from build123d import *

# Parameters (mm, degrees)
SKETCH1_R           = 3.4
SKETCH1_R_2         = 2.1
BOSS_EXTRUDE1_DEPTH = 205
FILLET1_R           = 2


with BuildPart() as part:
    # Sketch1 → Boss-Extrude1 (new body)
    with BuildSketch(Plane.XY):
        Polygon((15, -15), (4, -15), (4, -13), (8.25, -13), (8.25, -9.664213562), (4.585786438, -6), (-4.585786438, -6), (-8.25, -9.664213562), (-8.25, -13), (-4, -13), (-4, -15), (-15, -15), (-15, -4), (-13, -4), (-13, -8.25), (-9.664213562, -8.25), (-6, -4.585786438), (-6, 4.585786438), (-9.664213562, 8.25), (-13, 8.25), (-13, 4), (-15, 4), (-15, 15), (-4, 15), (-4, 13), (-8.25, 13), (-8.25, 9.664213562), (-4.585786438, 6), (4.585786438, 6), (8.25, 9.664213562), (8.25, 13), (4, 13), (4, 15), (15, 15), (15, 4), (13, 4), (13, 8.25), (9.664213562, 8.25), (6, 4.585786438), (6, -4.585786438), (9.664213562, -8.25), (13, -8.25), (13, -4), (15, -4), align=None)
        with Locations(Location((0, 0, 0), (0, 0, 180))):
            Circle(SKETCH1_R, mode=Mode.SUBTRACT)
        with Locations(Location((-11.6, 11.6, 0), (0, 0, 180))):
            Circle(SKETCH1_R_2, mode=Mode.SUBTRACT)
        with Locations(Location((11.6, 11.6, 0), (0, 0, 180))):
            Circle(SKETCH1_R_2, mode=Mode.SUBTRACT)
        with Locations(Location((11.6, -11.6, 0), (0, 0, 180))):
            Circle(SKETCH1_R_2, mode=Mode.SUBTRACT)
        with Locations(Location((-11.6, -11.6, 0), (0, 0, 180))):
            Circle(SKETCH1_R_2, mode=Mode.SUBTRACT)
    extrude(amount=BOSS_EXTRUDE1_DEPTH)

    # Fillet1
    fillet1_edges = [part.edges().sort_by_distance(p)[0] for p in [
        (-15, -15, 102.5),
        (-15, 15, 102.5),
        (15, 15, 102.5),
        (15, -15, 102.5),
    ]]
    fillet(fillet1_edges, radius=FILLET1_R)


solid = part.part
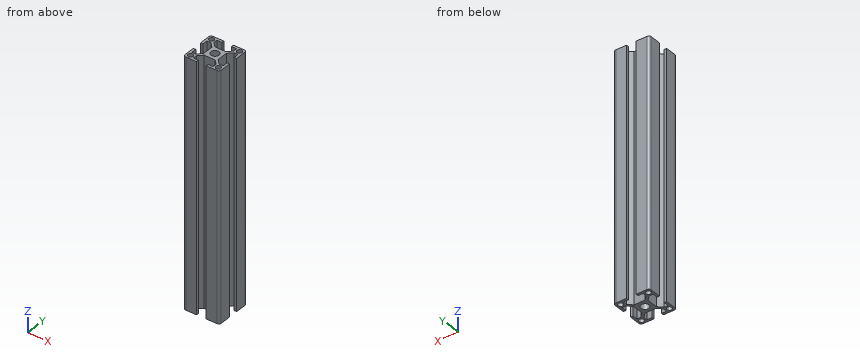
Geometry check sheet. Reference: the model listing, model coordinates, mm. Coordinates: 2 decimals unless noted, no trailing zeros. Loops run counter-clockwise (first coordinate to the right, second up) from the corner with the lowest first, then second, coordinate; pieces in that order, holes last. Notation, with made-up numbers: (70, -19.5) - (83, -19.5) arc R16 cw to (83, -9.5) - close; hole circle Ø5 at (5, -36.75). An arc over 180 degrees is marked (long way). Use one line per item in the form item = value. Start each with the question number.
Item 1: Section check B-B, the plane z = 118. Give the number of separate pieces and of enclosed holes in the cut face, and give its area (3 significant figures).
Item 2: Thickness scan on probe 1 along Y at (x, z) = (11.6, 50.5); probe 2 along Y at (x, z) = (4.25, 155). Record the ranges inside material, lowest first.
Item 3: Gauge pin test, flat ends, axial feed: pin 1 (1 mm diameter, centred on y = 14.5, z = 66, fed in from -X); pin 2 (5 mm diameter, centred on y = -2.5, z = 171, fed in from -X); pin 3 (3 mm diameter, centred on x = 0.5, z = 126, fed in from +Y); pin 4 (1 mm diameter, centred on x = -14.5, z = 89, fed in from +Y). Record the tip position at first contact, or that the pin passes through.
Item 4: Section check A-A, the plane x = 0. Enter the section's corners in (y, z).
Computed:
q1.separate_pieces = 1
q1.enclosed_holes = 5
q1.area = 333 mm2
q2.probe_1 = -15 to -13.7, -9.5 to -8.25, 8.25 to 9.5, 13.7 to 15
q2.probe_2 = -15 to -13, -6 to 6, 13 to 15
q3.pin_1 = -14.73
q3.pin_2 = -15
q3.pin_3 = 6
q3.pin_4 = 14.73
q4.outline = (-6, 0) - (-3.4, 0) - (-3.4, 205) - (-6, 205) - close; (3.4, 0) - (6, 0) - (6, 205) - (3.4, 205) - close
